The model under review builds one solid part; all positions refer to its coordinate system, in mm. A direction names the side the tool comes from. Round coordinates to 2 decimals unless told otherwise and drop trailing zeros. Write each loop counter-clockwise with the first axis right and the second up, starting at its lowest first coordinate (ties: lowest second). Pieces come first, ordered by that corner, then holes. Notation, with made-up numbers: (-36, 31.5) - (-9, 31.5) arc R5 cw to (-9, 37.5) - close; hole circle Ø10 at (12.5, 77.5). An arc over 180 degrees is marked (long way). Use one line per item in the form item = value.
from build123d import *

# Parameters (mm, degrees)
SKETCH1_R               = 2.4892
BOSS_EXTRUDE1_DEPTH     = 6.35
BOSS_EXTRUDE2_START     = -6.35
BOSS_EXTRUDE2_DEPTH     = 19.05
BOSS_EXTRUDE2_START_2   = -6.555460136
BOSS_EXTRUDE2_2_DEPTH   = 19.460920272
BOSS_EXTRUDE2_START_3   = -10
BOSS_EXTRUDE2_3_DEPTH   = 3.65
CUT_EXTRUDE1_DEPTH      = 27.910448217
CUT_EXTRUDE1_DEPTH_BACK = 27.910448217
SKETCH3_W               = 2.179354936
SKETCH3_H               = 6.35
CUT_EXTRUDE2_DEPTH      = 31.98795935
CUT_EXTRUDE2_DEPTH_BACK = 31.98795935


with BuildPart() as part:
    # Sketch1 → Boss-Extrude1 (new body)
    with BuildSketch(Plane(origin=(0, 0, 0), x_dir=(1, 0, 0), z_dir=(0, 1, 0))):
        with BuildLine():
            Line((9.525, -17.889269346), (-0.578271622, -16.817120786))
            Line((-0.578271622, -16.817120786), (-6.35, 0))
            Line((-6.35, 0), (12.7, 0))
            Line((12.7, 0), (12.7, -6.35))
            ThreePointArc((12.7, -6.35), (15.186560179, -13.240601753), (9.525, -17.889269346))
        make_face()
        with Locations(Location((9.525, -11.43, 0), (0, 0, 270))):
            Circle(SKETCH1_R, mode=Mode.SUBTRACT)
    extrude(amount=BOSS_EXTRUDE1_DEPTH)

    # Boss-Extrude2: read off the stored shape, not the designer's step
    # Boss-Extrude2 outline → Boss-Extrude2 (add)
    with BuildSketch(Plane.YZ.offset(BOSS_EXTRUDE2_START)):
        with BuildLine():
            ThreePointArc((11.551615481, -6.35), (12.905510296, -4.996105185), (11.551615481, -3.642210371))
            Line((11.551615481, -3.642210371), (6.35, 0))
            Line((6.35, 0), (0, 0))
            Line((0, 0), (-5.201615481, -3.642210371))
            ThreePointArc((-5.201615481, -3.642210371), (-6.555510296, -4.996105185), (-5.201615481, -6.35))
            Line((-5.201615481, -6.35), (11.551615481, -6.35))
        make_face()
    extrude(amount=BOSS_EXTRUDE2_DEPTH)

    # Boss-Extrude2 2 outline → Boss-Extrude2 2 (add)
    with BuildSketch(Plane(origin=(0, 0, 0), x_dir=(1, 0, 0), z_dir=(0, 1, 0)).offset(BOSS_EXTRUDE2_START_2)):
        Polygon((-8.529354936, 6.35), (-6.35, 0), (-6.35, 6.35), align=None)
    extrude(amount=BOSS_EXTRUDE2_2_DEPTH)

    # Boss-Extrude2 3 outline → Boss-Extrude2 3 (cut)
    with BuildSketch(Plane.YZ.offset(BOSS_EXTRUDE2_START_3)):
        with BuildLine():
            Line((12.905460136, 0), (6.35, 0))
            Line((6.35, 0), (11.551615481, -3.642210371))
            ThreePointArc((11.551615481, -3.642210371), (12.504834401, -4.034645431), (12.905460136, -4.984450993))
            Line((12.905460136, -4.984450993), (12.905460136, 0))
        make_face()
        with BuildLine():
            ThreePointArc((12.905460136, -5.007759378), (12.504834401, -5.95756494), (11.551615481, -6.35))
            Line((11.551615481, -6.35), (12.905460136, -6.35))
            Line((12.905460136, -6.35), (12.905460136, -5.007759378))
        make_face()
        with BuildLine():
            Line((0, 0), (-6.555460136, 0))
            Line((-6.555460136, 0), (-6.555460136, -4.984450993))
            ThreePointArc((-6.555460136, -4.984450993), (-6.154834401, -4.034645431), (-5.201615481, -3.642210371))
            Line((-5.201615481, -3.642210371), (0, 0))
        make_face()
        with BuildLine():
            ThreePointArc((-5.201615481, -6.35), (-6.154834401, -5.95756494), (-6.555460136, -5.007759378))
            Line((-6.555460136, -5.007759378), (-6.555460136, -6.35))
            Line((-6.555460136, -6.35), (-5.201615481, -6.35))
        make_face()
    extrude(amount=BOSS_EXTRUDE2_3_DEPTH, mode=Mode.SUBTRACT)

    # Sketch3 → Cut-Extrude1 (cut, two sides: drawn at the far end of the back side and taken through both)
    with BuildSketch(Plane.XZ.offset(-CUT_EXTRUDE1_DEPTH_BACK)):
        with Locations((-7.439677468, -3.175)):
            Rectangle(SKETCH3_W, SKETCH3_H)
    extrude(amount=CUT_EXTRUDE1_DEPTH + CUT_EXTRUDE1_DEPTH_BACK, mode=Mode.SUBTRACT)

    # Sketch4 → Cut-Extrude2 (cut, two sides: drawn at the far end of the back side and taken through both)
    with BuildSketch(Plane.ZY.offset(6.35).offset(-CUT_EXTRUDE2_DEPTH_BACK)):
        with BuildLine():
            ThreePointArc((-5.842, -4.417095512), (-5.087595278, -5.071775822), (-4.333190556, -4.417095512))
            Line((-4.333190556, -4.417095512), (-1.240306982, 0))
            Line((-1.240306982, 0), (0, 0))
            Line((0, 0), (-3.642210371, -5.201615481))
            ThreePointArc((-3.642210371, -5.201615481), (-4.996105185, -6.555510296), (-6.35, -5.201615481))
            Line((-6.35, -5.201615481), (-6.35, 11.551615481))
            ThreePointArc((-6.35, 11.551615481), (-4.996105185, 12.905510296), (-3.642210371, 11.551615481))
            Line((-3.642210371, 11.551615481), (0, 6.35))
            Line((0, 6.35), (-1.240306982, 6.35))
            Line((-1.240306982, 6.35), (-4.333190556, 10.767095512))
            ThreePointArc((-4.333190556, 10.767095512), (-5.087595278, 11.636415201), (-5.842, 10.767095512))
            Line((-5.842, 10.767095512), (-5.842, -4.417095512))
        make_face()
    extrude(amount=CUT_EXTRUDE2_DEPTH + CUT_EXTRUDE2_DEPTH_BACK, mode=Mode.SUBTRACT)


solid = part.part
(1) The part is to be moulded in two halves that separate along X. For faces 1 (the cylindrical face through (11.993, 3.131, 11.106)), 2 (the flat face through (4.54, 3.13, 17.36)), 3 (the flat face through (5, 0, 8)), say which applies: +X half, -X half, draft (parallel to the pull), parting line (faces both ways), or undercut.
Geometry results:
face_1 = undercut
face_2 = -X half
face_3 = draft
(2) Machinability: for faces 4 (the flat face through (12.7, 3, -1)), 5 (the flat face through (5, 6.35, 8)), 6 (the flat face through (-6.35, 3, -4)), which of the approach directions +Z, -Z, +X, -X, +Y, -Y give a long, thin tool a straight path to every point of the face, cutting with its end or side? Answer none if there is none.
Geometry results:
face_4 = -Z, +X, +Y, -Y
face_5 = +Z, +X, -X, +Y
face_6 = +Z, -Z, -X, +Y, -Y
(3) Add section A-A on y = 4.5. Write out the cut boundary in (x, z) (3 decimals), then the cut area to 3 significant figures.
Geometry results:
outline = (-6.35, -5.842) - (12.7, -5.842) - (12.7, 6.35) arc R6.35 ccw to (9.525, 17.889) - (-0.578, 16.817) - (-6.35, 0) - close; hole circle Ø4.978 at (9.525, 11.43)
area = 391 mm2
(4) Insertion check: P1, Ø3, axis at x = 9.525, z = 11.43, coming from the -Y side; P2, Ø7.5, axis at x = 6, y = 5.5, coming from the -Z side; P3, Ø1.5, axis at x = -1, z = -2, coming from the -Y side; P4, Ø2, axis at y = 7, z = 10.5, coming from the +X side. Each pin has a flat end and moves straight along its axis. Give the tip position at first contact, or say it passes through.
Geometry results:
P1 = through
P2 = -5.84
P3 = -2.16
P4 = 15.41
(5) To check wall thickness, follow L1, parallel to Y at x = -2, z = 10; L2, parallel to X at y = 4.25, z = 9.5. State the ranges of each line that lie inside material, in increasing order.
Geometry results:
L1 = 0 to 6.35
L2 = -3.09 to 7.95, 11.1 to 15.07
(6) Add section D-D on x = 1.25. Write out the cut boundary in (y, z), then the cut area to 3 significant figures.
Geometry results:
outline = (-4.42, -5.84) - (10.77, -5.84) arc R0.76 ccw (long way) to (10.77, -4.33) - (6.35, -1.24) - (6.35, 17.01) - (0, 17.01) - (0, -1.24) - (-4.42, -4.33) arc R0.76 ccw to start
area = 174 mm2
(7) Add section C-C on z = 11.43. Write out the cut boundary in (x, y).
Geometry results:
outline = (-2.43, 0) - (7.04, 0) - (7.04, 6.35) - (-2.43, 6.35) - close; (12.01, 0) - (15.41, 0) - (15.41, 6.35) - (12.01, 6.35) - close
(8) Add section B-B on x = 7.5. Write out the cut boundary in (y, z), then the cut area to 3 significant figures.
Geometry results:
outline = (-4.42, -5.84) - (10.77, -5.84) arc R0.76 ccw (long way) to (10.77, -4.33) - (6.35, -1.24) - (6.35, 9.98) - (0, 9.98) - (0, -1.24) - (-4.42, -4.33) arc R0.76 ccw to start; (0, 12.88) - (6.35, 12.88) - (6.35, 17.67) - (0, 17.67) - close
area = 160 mm2
